Geometry check sheet. Reference: the model listing, model coordinates, mm. Give positions to 0.01 mm unless a question says otherwise; leave off trailing zeros. Loops run counter-clockwise (first coordinate to the right, second up) from the corner with the lowest first, then second, coordinate; pieces in that order, holes last. Notation, with made-up numbers: (-39.75, 66.5) -> (14.25, 66.5) arc R21 cw to (14.25, 96.5) -> close; hole circle Ø7 at (-38, -25.75). An arc over 180 degrees is marked (long way). Write item = value, one per line. Start each with the question number.
```python
from build123d import *

# Parameters (mm, degrees)
SKETCH1_R           = 2.8
SKETCH1_R_2         = 4.9
SKETCH1_R_3         = 1.6
BOSS_EXTRUDE1_DEPTH = 3.175
CUT_EXTRUDE1_REACH  = 5.175
SKETCH3_R           = 1.6


with BuildPart() as part:
    # Sketch1 → Boss-Extrude1 (new body)
    with BuildSketch(Plane(origin=(0, 0, 0), x_dir=(1, 0, 0), z_dir=(0, 1, 0))):
        with BuildLine():
            Line((12.18, 33), (12.18, 22.7))
            ThreePointArc((12.18, 22.7), (9.251067812, 15.628932188), (2.18, 12.7))
            Line((2.18, 12.7), (0, 12.7))
            ThreePointArc((0, 12.7), (-10.837940978, -6.620350093), (11.29936434, -5.797789709))
            ThreePointArc((11.29936434, -5.797789709), (15.26781807, -0.83060398), (20.857391991, 2.198954148))
            ThreePointArc((20.857391991, 2.198954148), (29.041537075, 7.982602032), (32.18, 17.5))
            Line((32.18, 17.5), (32.18, 33))
            ThreePointArc((32.18, 33), (22.18, 43), (12.18, 33))
        make_face()
        with Locations((22.18, 17.5)):
            Circle(SKETCH1_R, mode=Mode.SUBTRACT)
        with Locations((22.18, 33)):
            Circle(SKETCH1_R, mode=Mode.SUBTRACT)
        Circle(SKETCH1_R_2, mode=Mode.SUBTRACT)
        with Locations((-8.25, 0)):
            Circle(SKETCH1_R_3, mode=Mode.SUBTRACT)
        with Locations((4.125, 7.144709581)):
            Circle(SKETCH1_R_3, mode=Mode.SUBTRACT)
        with Locations((4.125, -7.144709581)):
            Circle(SKETCH1_R_3, mode=Mode.SUBTRACT)
    extrude(amount=BOSS_EXTRUDE1_DEPTH)

    # Sketch3 → Cut-Extrude1 (cut, up to next)
    with BuildSketch(Plane(origin=(0, 3.175, 0), x_dir=(1, 0, 0), z_dir=(0, 1, 0)), mode=Mode.PRIVATE) as cut_extrude1_sk1:
        with Locations((9.526279442, 0)):
            Circle(SKETCH3_R)
    cut_extrude1_tool1 = extrude(cut_extrude1_sk1.sketch, amount=-CUT_EXTRUDE1_REACH, mode=Mode.PRIVATE) & part.part
    add(cut_extrude1_tool1.solids().sort_by_distance((9.526279, 3.175, 0))[0], mode=Mode.SUBTRACT)
    # Sketch3 → Cut-Extrude1 (cut, up to next)
    with BuildSketch(Plane(origin=(0, 3.175, 0), x_dir=(1, 0, 0), z_dir=(0, 1, 0)), mode=Mode.PRIVATE) as cut_extrude1_sk2:
        with Locations((-4.763139721, -8.25)):
            Circle(SKETCH3_R)
    cut_extrude1_tool2 = extrude(cut_extrude1_sk2.sketch, amount=-CUT_EXTRUDE1_REACH, mode=Mode.PRIVATE) & part.part
    add(cut_extrude1_tool2.solids().sort_by_distance((-4.76314, 3.175, 8.25))[0], mode=Mode.SUBTRACT)
    # Sketch3 → Cut-Extrude1 (cut, up to next)
    with BuildSketch(Plane(origin=(0, 3.175, 0), x_dir=(1, 0, 0), z_dir=(0, 1, 0)), mode=Mode.PRIVATE) as cut_extrude1_sk3:
        with Locations((-4.763139721, 8.25)):
            Circle(SKETCH3_R)
    cut_extrude1_tool3 = extrude(cut_extrude1_sk3.sketch, amount=-CUT_EXTRUDE1_REACH, mode=Mode.PRIVATE) & part.part
    add(cut_extrude1_tool3.solids().sort_by_distance((-4.76314, 3.175, -8.25))[0], mode=Mode.SUBTRACT)


solid = part.part
```
1) Section check D-D (z = -28). Enter the section's corners in (x, y) (3 decimals).
2) Section check C-C (y = 1.2). Give the number of separate pieces and of enclosed holes in the cut face, plus the area to 3 significant figures.
3) Section check A-A (x = 20). Enter the section's corners in (y, z) (3 decimals), plus the area to 3 significant figures.
4) Draft check along Z on faces 1 (the cylindrical face through (23.472, 1.565, -15.016)), 2 (the flat face through (1, 2, -12.7)), 3 (the flat face through (12.18, 2, -28)). Enter one of: released by +Z, released by -Z, zero draft, split by the parting line, or undercut.
5) Thickness scan on line 1 (X direction, y = 0.75, z = 0); line 2 (Z direction, x = 24, y = 0.35); line 3 (X direction, y = 1.3, z = 7). Record the ranges inside material, lowest first.
6) Section check B-B (x = 8.5). Enter the section's corners in (y, z) (1 decimal), plus the area to 3 significant figures.
7) Depth check by flat-ended pin: pin 1 Ø1.5 at (x, y) = (4.5, 2) entering from +Z; pin 2 Ø9 at (x, z) = (0, 0) entering from -Y; pin 3 Ø1.6 at (y, z) = (2.5, -25.5) entering from -X; pin 4 Ø1.1 at (x, y) = (1.5, 2) entering from -Z. Enter the tip coordinate at first touch or a pass-through.
Check result:
q1.outline = (12.18, 0) -> (32.18, 0) -> (32.18, 3.175) -> (12.18, 3.175) -> close
q2.separate_pieces = 1
q2.enclosed_holes = 9
q2.area = 1,130 mm2
q3.outline = (0, -42.759) -> (3.175, -42.759) -> (3.175, -34.757) -> (0, -34.757) -> close; (0, -31.243) -> (3.175, -31.243) -> (3.175, -19.257) -> (0, -19.257) -> close; (0, -15.743) -> (3.175, -15.743) -> (3.175, -1.91) -> (0, -1.91) -> close
q3.area = 107 mm2
q4.face_1 = undercut
q4.face_2 = released by -Z
q4.face_3 = zero draft
q5.line_1 = -12.7 to -9.85, -6.65 to -4.9, 4.9 to 7.93, 11.13 to 16.35
q5.line_2 = -42.83 to -35.13, -30.87 to -19.63, -15.37 to -3.54
q5.line_3 = -10.6 to -5.76, -3.76 to 2.53, 5.72 to 10.6
q6.outline = (0, -15) -> (3.2, -15) -> (3.2, -1.2) -> (0, -1.2) -> close; (0, 1.2) -> (3.2, 1.2) -> (3.2, 9.4) -> (0, 9.4) -> close
q6.area = 69.6 mm2
q7.pin_1 = 12.13
q7.pin_2 = through
q7.pin_3 = 12.18
q7.pin_4 = -12.7
